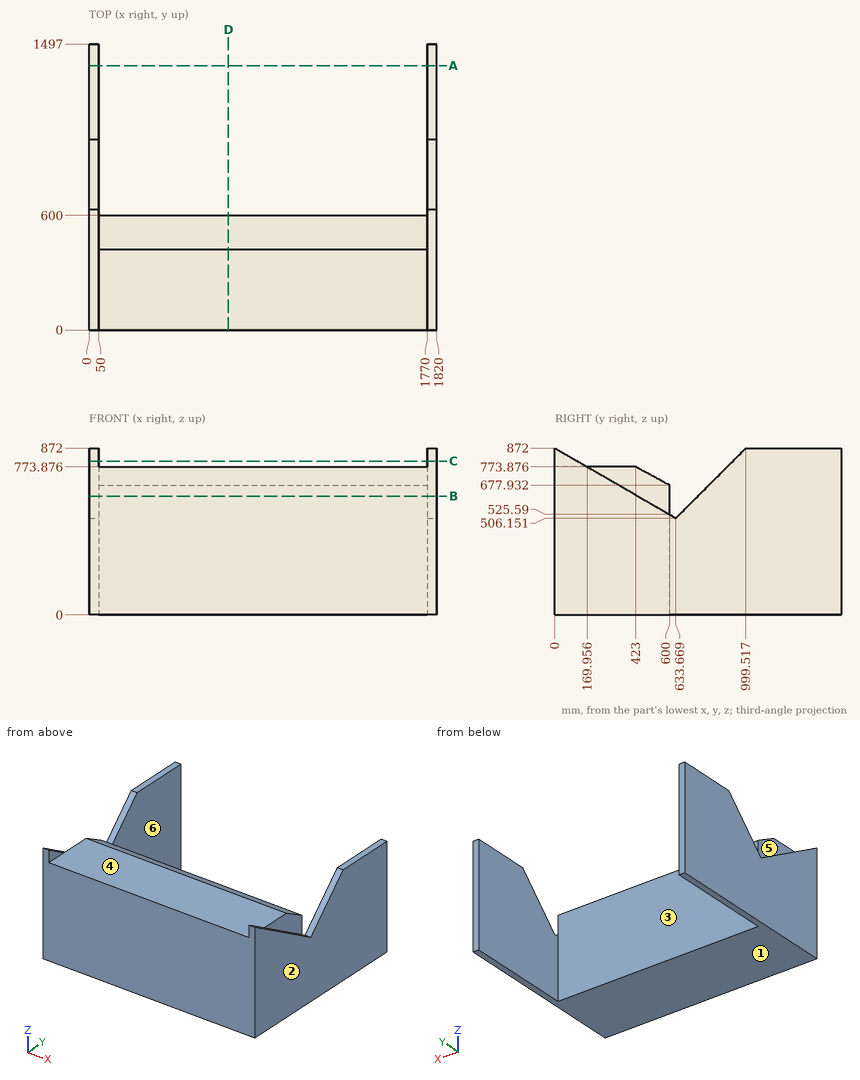
Input: dimensioned drawing with shaded views. Units: mm. Origin: part minimum x, y, z. A direction names the side the tool comes from. Coordinates: 2 decimals unless noted, no trailing zeros. Loops run counter-clockwise (first coordinate to the right, second up) from the corner with the lowest first, then second, coordinate; pieces in that order, holes last. Notation, with made-up numbers: M -32.5,60.5 L 0.5,60.5 A21 ccw 0.5,75.5 Z; hole C 88,-30 d8. An arc over 180 degrees is marked long. Use a Markdown table: item, result. Add a question column.
1) Section A-A, the plane y = 1384. Return the cut outline in (x, z).
2) Section B-B, the plane z = 621. Return the cut outline in (x, y) (1 decimal), plus the area to 3 significant figures.
3) Section C-C, the plane z = 804.5. Return the cut outline in (x, y).
4) Section D-D, the plane x = 729. Return the cut outline in (y, z) (1 decimal).
5) Line query: L1, parallel to X at y = 790, z = 178.5; L2, parallel to Z at x = 617, y = 278 (1 decimal); L3, parallel to Y at x = 658, z = 169. Output: solid intervals per line, ascending. Write a range as from..to.
6) Pin query (flat end, axial travel): P1, Ø6, axis at x = 699, z = 708, coming from the +Y side (1 decimal); P2, Ø2, axis at x = 1550.5, z = 488, coming from the +Y side; P3, Ø4, axis at x = 1399.5, z = 727, coming from the +Y side (1 decimal). Return the tip coordinate at first contact, or that it passes through.
7) Draft query along X for the marked faces 1, 2 and 3. Return one class per face: +X half, -X half, draft (parallel to the pull), parting line (faces both ways), or undercut.
8) Set-up query: the marked faces 4, 5 and 6. Return all of +Z, -Z, +X, -X, +Y, -Y with unobstructed straight access to the full face (end or side cutting, diameter ignored); none if empty.
Answer below:
| question | item | result |
|---|---|---|
| 1 | outline | M 0,0 L 50,0 L 50,872 L 0,872 Z; M 1770,0 L 1820,0 L 1820,872 L 1770,872 Z |
| 2 | outline | M 0,0 L 1820,0 L 1820,434.7 L 1770,434.7 L 1770,600 L 50,600 L 50,434.7 L 0,434.7 Z; M 0,748.5 L 50,748.5 L 50,1497 L 0,1497 Z; M 1770,748.5 L 1820,748.5 L 1820,1497 L 1770,1497 Z |
| 2 | area | 1,150,000 mm2 |
| 3 | outline | M 0,0 L 50,0 L 50,116.91 L 0,116.91 Z; M 0,932.02 L 50,932.02 L 50,1497 L 0,1497 Z; M 1770,0 L 1820,0 L 1820,116.91 L 1770,116.91 Z; M 1770,932.02 L 1820,932.02 L 1820,1497 L 1770,1497 Z |
| 4 | outline | M 0,0 L 600,0 L 600,677.9 L 423,773.9 L 0,773.9 Z |
| 5 | L1 | 0..50, 1770..1820 |
| 5 | L2 | 0..773.9 |
| 5 | L3 | 0..600 |
| 6 | P1 | y = 550.1 |
| 6 | P2 | y = 600 |
| 6 | P3 | y = 513.2 |
| 7 | face 1 | draft |
| 7 | face 2 | +X half |
| 7 | face 3 | undercut |
| 8 | face 4 | +Z, +Y, -Y |
| 8 | face 5 | +Z, -X |
| 8 | face 6 | +Z, -Z, +Y |
